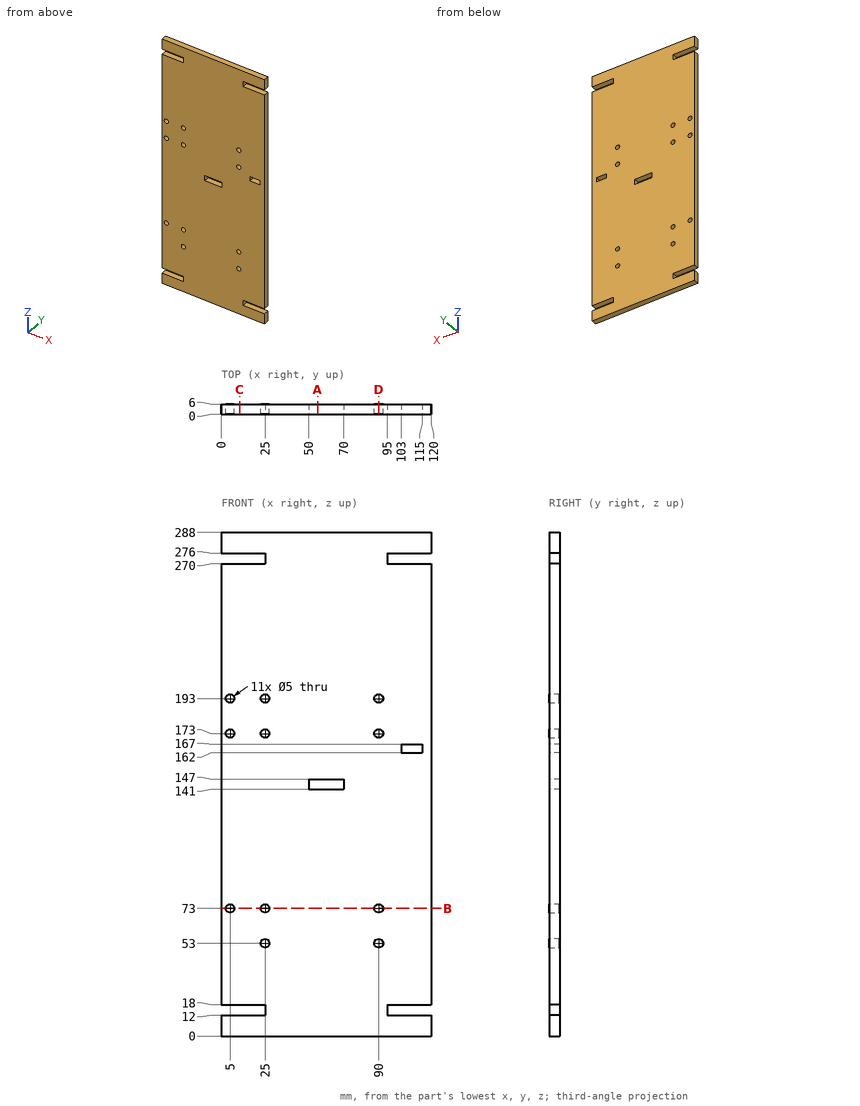
Answer from the drawing. Dimensions are ordinates in mm from the lowest x, y and z of the part. Round coordinates to 2 decimals unless told otherwise and drop trailing zeros. Order: outer loops, then holes, each group sorted by start corner. A loop starts at its lowest first (then second) coordinate and runs counter-clockwise, first axis right, second up. Notation, with made-up numbers: (-27, 63.25) - (-4, 63.25) arc R19 ccw to (-4, 87.25) - close; hole circle Ø9 at (-8, -21). An arc over 180 degrees is marked (long way). Put each result on its own line as item: value. Start each with the question number.
(1) Find section A-A (x = 55). Give the vertices of the cut face in (y, z), plus the area to 3 significant figures.
(2) Given P1, Ø1.8, axis at y = 1.5, z = 13.5, coming from the -X side; P2, Ø1.8, axis at y = 4, z = 271.5, coming from the +X side, each flat-ended and moving along its own axis, determine where each tip first touches the part or whether it passes through.
(3) Find section C-C (x = 10.5). Give the vertices of the cut face in (y, z).
(4) Find section B-B (z = 73). Give the vertices of the cut face in (x, y), plus the area to 3 significant figures.
(5) Find section D-D (x = 90). Give the vertices of the cut face in (y, z).
(6) Straight lines are drawn through the part: probe 1 along X at (y, z) = (1.55, 53); probe 2 along X at (y, z) = (2.25, 73); probe 3 along Z at (x, y) = (22, 0.3). For each, find the intervals that lie inside material, in ascending order. Write a range as from..to.
Reply:
1. outline: (0, 0) - (6, 0) - (6, 141) - (0, 141) - close; (0, 147) - (6, 147) - (6, 288) - (0, 288) - close
1. area: 1,690 mm^2
2. P1: x = 25
2. P2: x = 95
3. outline: (0, 0) - (6, 0) - (6, 12) - (0, 12) - close; (0, 18) - (6, 18) - (6, 270) - (0, 270) - close; (0, 276) - (6, 276) - (6, 288) - (0, 288) - close
4. outline: (0, 0) - (2.5, 0) - (2.5, 6) - (0, 6) - close; (7.5, 0) - (22.5, 0) - (22.5, 6) - (7.5, 6) - close; (27.5, 0) - (87.5, 0) - (87.5, 6) - (27.5, 6) - close; (92.5, 0) - (120, 0) - (120, 6) - (92.5, 6) - close
4. area: 630 mm^2
5. outline: (0, 0) - (6, 0) - (6, 50.5) - (0, 50.5) - close; (0, 55.5) - (6, 55.5) - (6, 70.5) - (0, 70.5) - close; (0, 75.5) - (6, 75.5) - (6, 170.5) - (0, 170.5) - close; (0, 175.5) - (6, 175.5) - (6, 190.5) - (0, 190.5) - close; (0, 195.5) - (6, 195.5) - (6, 288) - (0, 288) - close
6. probe 1: 0..22.5, 27.5..87.5, 92.5..120
6. probe 2: 0..2.5, 7.5..22.5, 27.5..87.5, 92.5..120
6. probe 3: 0..12, 18..270, 276..288
